```python
from build123d import *

# Parameters (mm, degrees)
SKETCH1_R           = 30
BOSS_EXTRUDE1_DEPTH = 6
SKETCH6_R           = 2.77
BOSS_EXTRUDE3_DEPTH = 7.5
CIRPATTERN3_COUNT   = 4
SKETCH11_W          = 10
SKETCH11_H          = 10
CUT_EXTRUDE3_DEPTH  = 3


with BuildPart() as part:
    # Sketch1 → Boss-Extrude1 (new body)
    with BuildSketch(Plane(origin=(0, 0, 0), x_dir=(1, 0, 0), z_dir=(0, 1, 0))):
        with Locations(Location((0, 0, 0), (0, 0, 270))):
            Circle(SKETCH1_R)
    extrude(amount=BOSS_EXTRUDE1_DEPTH)

    # Sketch6 → Boss-Extrude3 (add)
    with BuildSketch(Plane(origin=(0, 0, -4.132474232), x_dir=(1, 0, 0), z_dir=(0, -1, 0))):
        with Locations(Location((-0.002388639, 27.198186003, 0), (0, 0, 90))):
            Circle(SKETCH6_R)
        Polygon((2.047611361, 27.873186003), (2.047611361, 26.523186003), (0.672611361, 26.523186003), (0.672611361, 25.148186003), (-0.677388639, 25.148186003), (-0.677388639, 26.523186003), (-2.052388639, 26.523186003), (-2.052388639, 27.873186003), (-0.677388639, 27.873186003), (-0.677388639, 29.248186003), (0.672611361, 29.248186003), (0.672611361, 27.873186003), align=None, mode=Mode.SUBTRACT)
    boss_extrude3 = extrude(amount=BOSS_EXTRUDE3_DEPTH)

    # CirPattern3: Boss-Extrude3 ×4 about axis
    cirpattern3_axis = Axis((2.0539e-05, 0, -0.19833635), (0, 1, 0))
    for i in range(1, CIRPATTERN3_COUNT):
        add(boss_extrude3.rotate(cirpattern3_axis, i * 360 / CIRPATTERN3_COUNT))

    # Sketch11 → Cut-Extrude3 (cut)
    with BuildSketch(Plane(origin=(0, 6, 0), x_dir=(1, 0, 0), z_dir=(0, 1, 0))):
        Rectangle(SKETCH11_W, SKETCH11_H)
    extrude(amount=-CUT_EXTRUDE3_DEPTH, mode=Mode.SUBTRACT)


solid = part.part
```
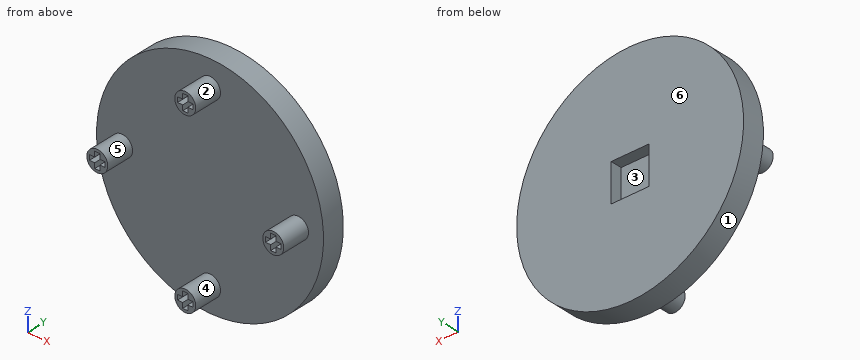
Part model, mm, in its own coordinate system. Face numbers are marked on the shaded views. A direction names the side the tool comes from. Round coordinates to 2 decimals unless told otherwise and drop trailing zeros. Order: outer loops, then holes, each group sorted by start corner. A loop starts at its lowest first (then second) coordinate and runs counter-clockwise, first axis right, second up. Notation, with made-up numbers: M 66.25,-19.5 L 73.25,-19.5 A18 ccw 73.25,3.5 Z; hole C -33.5,53 d3. An arc over 180 degrees is marked long. Put each result on its own line as item: value. Start each with the question number.
1. Slice it at C-C on x = -15.5. List the corners of the cut face in (y, z).
2. Two-plate mould, pull along Z, no slides. Class the marked faces 4, 5 and 6: +Z half, -Z half, draft (parallel to the pull), parting line (faces both ways), or undercut.
3. Slice it at D-D on y = -3.25. State how many separate pieces and enclosed holes the cut face has, then the cut area to 3 significant figures.
4. Tool access for the marked faces 1, 2 and 3: list every direction of +Z, -Z, +X, -X, +Y, -Y with a clear straight run to the whole face (end or side of a thin tool).
5. Slice it at B-B on y = 1. List the corners of the cut face in (x, z).
6. Slice it at A-A on y = 4.5. List the corners of the cut face in (x, z).
7. Drill centre lines: probe 1 along Y at (x, z) = (-6, 9); probe 2 along X at (y, z) = (-4.5, 24); probe 3 along X at (y, z) = (4.25, 24.5). Where is each one in solid material? Low to high. Write a range as [from, to].
8. Drop flat-ended pins along their axis: pin 1 (1.5 mm diameter, centred on y = -3.5, z = -25, fed in from +X); pin 2 (1.1 mm diameter, centred on y = -4, z = 0, fed in from -X); pin 3 (1.1 mm diameter, centred on y = -2, z = 1.5, fed in from +X); pin 4 (1.2 mm diameter, centred on x = -24, z = 0, fed in from -Y). Give the stop position or say it passes through.
Findings:
1. outline: M 0,-25.69 L 6,-25.69 L 6,25.69 L 0,25.69 Z
2. face 4: undercut
2. face 5: parting line
2. face 6: draft
3. separate pieces: 4
3. enclosed holes: 4
3. area: 59.4 mm2
4. face 1: +Y, -Y
4. face 2: -Y
4. face 3: +Y
5. outline: C 0,0 d60
6. outline: C 0,0 d60; hole M -5,-5 L 5,-5 L 5,5 L -5,5 Z
7. probe 1: [0, 6]
7. probe 2: [-2.61, -0.68], [0.67, 2.61]
7. probe 3: [-17.31, 17.31]
8. pin 1: x = 2.66
8. pin 2: x = -26.03
8. pin 3: x = 25.79
8. pin 4: y = -7.5
